Check sheet for the drawn part. Datum: minimum x, y, z corner. Units: mm. Round coordinates to 2 decimals unless told otherwise and drop trailing zeros. Write each loop counter-clockwise with the first axis right and the second up, starting at its lowest first coordinate (ties: lowest second). Pieces come first, ordered by that corner, then holes. Notation, with made-up numbers: M -26.75,57 L -10.75,57 A10 ccw -10.75,70 Z; hole C -21.75,61.25 d1. An arc over 180 degrees is marked long. One line per item, written item: value.
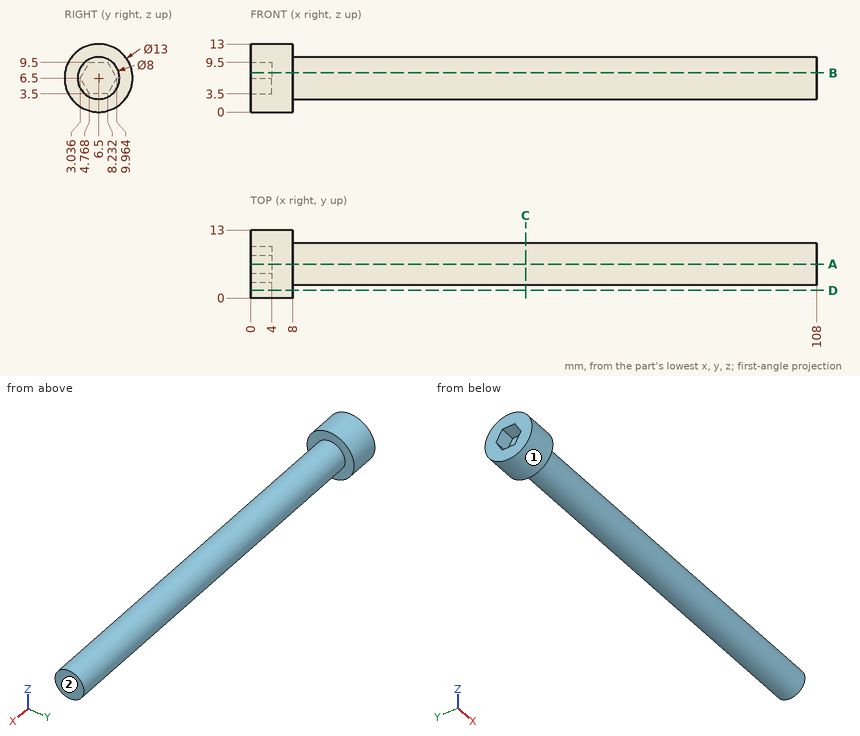
Q1. Draft check along X on the marked faces 1 and 2. Enter one of: pulls with the +X half, pulls with the -X half, needs draft (parallel to the pull), parting line crosses it, or undercut.
Completed:
face 1: needs draft
face 2: pulls with the +X half
Q2. Sectioned sample at D-D on y = 1.5. Enter the section's corners in (x, z).
Completed:
outline: M 0,2.35 L 8,2.35 L 8,10.65 L 0,10.65 Z
Q3. Scan lines: line 1 (X direction, y = 5.75, z = 10.5); line 2 (Z direction, x = 89.5, y = 8.5); line 3 (Z direction, x = 60, y = 6.75). Record each from-to range of solid material in increasing order. Write a range as [from, to].
Completed:
line 1: [0, 8]
line 2: [3.04, 9.96]
line 3: [2.51, 10.49]
Q4. Sectioned sample at A-A on y = 6.5. Enter the section's corners in (x, z).
Completed:
outline: M 0,0 L 8,0 L 8,2.5 L 108,2.5 L 108,10.5 L 8,10.5 L 8,13 L 0,13 L 0,9.5 L 4,9.5 L 4,3.5 L 0,3.5 Z
Q5. Depth check by flat-ended pin: P1, Ø1, axis at x = 2.5, y = 6, coming from the +Z side; P2, Ø3, axis at x = 94.5, z = 9.5, coming from the -Y side; P3, Ø1.5, axis at x = 48.5, y = 10, coming from the -Z side (1 decimal); P4, Ø4, axis at x = 56, z = 4, coming from the -Y side. Enter the tip coordinate at first touch or a pass-through.
Completed:
P1: z = 13
P2: y = 2.79
P3: z = 3.6
P4: y = 2.53
Q6. Sectioned sample at B-B on z = 7.5. Enter the section's corners in (x, y).
Completed:
outline: M 0,0.08 L 8,0.08 L 8,2.63 L 108,2.63 L 108,10.37 L 8,10.37 L 8,12.92 L 0,12.92 L 0,9.39 L 4,9.39 L 4,3.61 L 0,3.61 Z
Q7. Sectioned sample at C-C on x = 52.5. Enter the section's corners in (y, z).
Completed:
outline: C 6.5,6.5 d8
